Could you check a few things on this drawing? It's one solid part, dimensions in mm from its lowest x, y, z. Round coordinates to 2 decimals unless told otherwise and drop trailing zeros. Write each loop counter-clockwise with the first axis right and the second up, starting at its lowest first coordinate (ties: lowest second). Pieces come first, ordered by that corner, then holes. Notation, with made-up numbers: (47, 73) -> (56, 73) arc R17 cw to (56, 84) -> close; hole circle Ø6 at (-31, 30). An arc over 180 degrees is marked (long way). Answer in a Markdown table with one row per item.
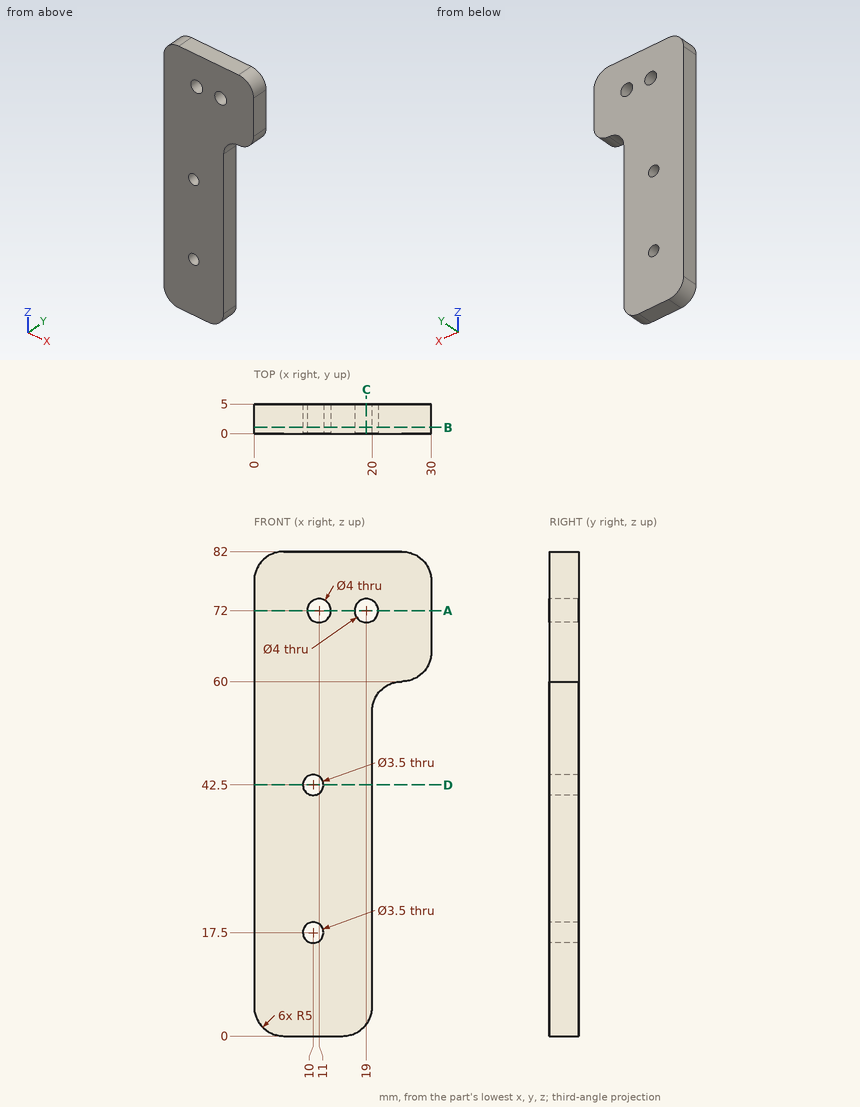
1) For pin 1 (1 mm diameter, centred on y = 2, z = 33.5, fed in from +X); pin 2 (1.5 mm diameter, centred on x = 17.5, y = 3.5, fed in from -Z), each with a flat end and sliding along its axis, tell me the tip position at first contact or that it passes through.
Response:
| item | result |
|---|---|
| pin 1 | stops at x = 20 |
| pin 2 | stops at z = 0.32 |
2) I want a section at C-C, the plane x = 19. List the corners of the cut face in (y, z) for me, and give its area (3 significant figures).
Response:
| item | result |
|---|---|
| outline | (0, 2) -> (5, 2) -> (5, 70) -> (0, 70) -> close; (0, 74) -> (5, 74) -> (5, 82) -> (0, 82) -> close |
| area | 380 mm^2 |
3) I want a section at A-A, the plane z = 72. List the corners of the cut face in (x, y) for me.
Response:
| item | result |
|---|---|
| outline | (0, 0) -> (9, 0) -> (9, 5) -> (0, 5) -> close; (13, 0) -> (17, 0) -> (17, 5) -> (13, 5) -> close; (21, 0) -> (30, 0) -> (30, 5) -> (21, 5) -> close |
4) I need wall thicknesses on line 1 (X direction, y = 2.35, z = 72); line 2 (X direction, y = 2.65, z = 42.5); line 3 (Z direction, x = 10, y = 3.8). Which ranges of each line are inside material? Lowest first, please. Write a range as [from, to].
Response:
| item | result |
|---|---|
| line 1 | x = [0, 9], [13, 17], [21, 30] |
| line 2 | x = [0, 8.25], [11.75, 20] |
| line 3 | z = [0, 15.75], [19.25, 40.75], [44.25, 70.27], [73.73, 82] |
5) I want a section at B-B, the plane y = 1.05. Count the separate pieces of the cut face and the enclosed holes in it, and give its area (3 significant figures).
Response:
| item | result |
|---|---|
| separate pieces | 1 |
| enclosed holes | 4 |
| area | 1,790 mm^2 |
6) I want a section at D-D, the plane z = 42.5. List the corners of the cut face in (x, y) for me.
Response:
| item | result |
|---|---|
| outline | (0, 0) -> (8.25, 0) -> (8.25, 5) -> (0, 5) -> close; (11.75, 0) -> (20, 0) -> (20, 5) -> (11.75, 5) -> close |
